from build123d import *

# Parameters (mm, degrees)
F0_R        = 15
F1_DEPTH    = 10.5
F3_R        = 0.75
F5_R        = 1
F6_T1_DEPTH = 20.8553390593


# Not quite as in the source:
# - a fillet or chamfer that OpenCascade refuses, or shapes differently, is made with other operations: its cross-section is extruded or revolved along the edge and cut away or added


with BuildPart() as f1:
    # F0 (on Top) → F1 (new body)
    with BuildSketch(Plane.XY):
        Polygon((-11.5, -19.5), (11.5, -19.5), (19.5, -11.5), (19.5, 11.5), (11.5, 19.5), (-11.5, 19.5), (-19.5, 11.5), (-19.5, -11.5), align=None)
        Circle(F0_R, mode=Mode.SUBTRACT)
    extrude(amount=F1_DEPTH)

    # F4: sweep along a path in F2
    with BuildLine(Plane.XY.offset(10.5)) as f4_path:
        Line((18.75, 11.1893398282), (18.75, -11.1893398282))
        Line((18.75, -11.1893398282), (11.1893398282, -18.75))
        Line((11.1893398282, -18.75), (-11.1893398282, -18.75))
        Line((-11.1893398282, -18.75), (-18.75, -11.1893398282))
        Line((-18.75, -11.1893398282), (-18.75, 11.1893398282))
        Line((-18.75, 11.1893398282), (-11.1893398282, 18.75))
        Line((-11.1893398282, 18.75), (11.1893398282, 18.75))
        Line((11.1893398282, 18.75), (18.75, 11.1893398282))
    # F3 (on Front) → F4 (sweep)
    with BuildSketch(Plane.XZ):
        with Locations((18.75, 10.5)):
            Circle(F3_R)
    sweep(path=f4_path.line, transition=Transition.RIGHT)

    # F5
    f5_edges = [f1.edges().sort_by_distance(p)[0] for p in [
        (18, 0, 10.5),
        (14.43934, -14.43934, 10.5),
        (0, -18, 10.5),
        (-14.43934, -14.43934, 10.5),
        (-18, 0, 10.5),
        (-14.43934, 14.43934, 10.5),
        (0, 18, 10.5),
        (14.43934, 14.43934, 10.5),
    ]]
    fillet(f5_edges, radius=F5_R)

    # F6: fillet of radius 5 on 8 edges, made by hand

    # F6_s2 → F6_t1 (cut)
    with BuildSketch(Plane.XY.offset(-5.1776695297)):
        with BuildLine():
            ThreePointArc((-18.0355339059, -12.9644660941), (-19.1193976626, -11.34234935), (-19.5, -9.4289321881))
            Line((-19.5, -9.4289321881), (-19.5, -11.5))
            Line((-19.5, -11.5), (-18.0355339059, -12.9644660941))
        make_face()
        with BuildLine():
            ThreePointArc((-9.4289321881, -19.5), (-11.34234935, -19.1193976626), (-12.9644660941, -18.0355339059))
            Line((-12.9644660941, -18.0355339059), (-11.5, -19.5))
            Line((-11.5, -19.5), (-9.4289321881, -19.5))
        make_face()
        with BuildLine():
            ThreePointArc((9.4289321881, -19.5), (11.34234935, -19.1193976626), (12.9644660941, -18.0355339059))
            Line((12.9644660941, -18.0355339059), (11.5, -19.5))
            Line((11.5, -19.5), (9.4289321881, -19.5))
        make_face()
        with BuildLine():
            ThreePointArc((18.0355339059, -12.9644660941), (19.1193976626, -11.34234935), (19.5, -9.4289321881))
            Line((19.5, -9.4289321881), (19.5, -11.5))
            Line((19.5, -11.5), (18.0355339059, -12.9644660941))
        make_face()
        with BuildLine():
            ThreePointArc((-9.4289321881, 19.5), (-11.34234935, 19.1193976626), (-12.9644660941, 18.0355339059))
            Line((-12.9644660941, 18.0355339059), (-11.5, 19.5))
            Line((-11.5, 19.5), (-9.4289321881, 19.5))
        make_face()
        with BuildLine():
            ThreePointArc((-19.5, 9.4289321881), (-19.1193976626, 11.34234935), (-18.0355339059, 12.9644660941))
            Line((-18.0355339059, 12.9644660941), (-19.5, 11.5))
            Line((-19.5, 11.5), (-19.5, 9.4289321881))
        make_face()
        with BuildLine():
            ThreePointArc((12.9644660941, 18.0355339059), (11.34234935, 19.1193976626), (9.4289321881, 19.5))
            Line((9.4289321881, 19.5), (11.5, 19.5))
            Line((11.5, 19.5), (12.9644660941, 18.0355339059))
        make_face()
        with BuildLine():
            ThreePointArc((19.5, 9.4289321881), (19.1193976626, 11.34234935), (18.0355339059, 12.9644660941))
            Line((18.0355339059, 12.9644660941), (19.5, 11.5))
            Line((19.5, 11.5), (19.5, 9.4289321881))
        make_face()
    extrude(amount=F6_T1_DEPTH, mode=Mode.SUBTRACT)


solid = f1.part
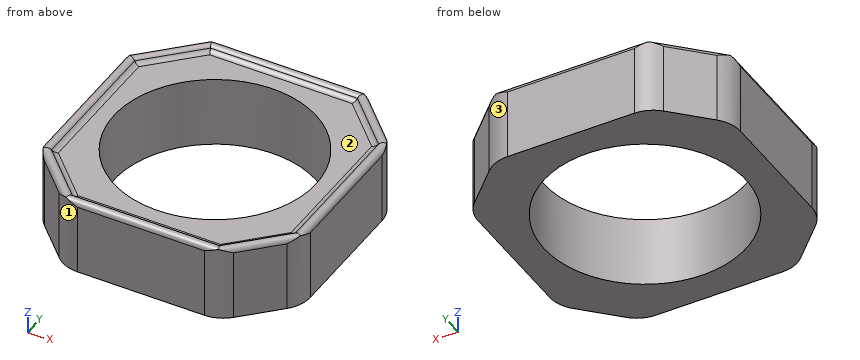
Source: CAD feature listing. Evaluate the final solid. Frame: model axes, mm. Face numbers are marked on the shaded views. Coordinates: 2 decimals unless noted, no trailing zeros. Loops run counter-clockwise (first coordinate to the right, second up) from the corner with the lowest first, then second, coordinate; pieces in that order, holes last. Notation, with made-up numbers: (-8.5, -33) -> (-3.5, -33) arc R30 ccw to (-3.5, 4) -> close; hole circle Ø2 at (30, -23.75). An arc over 180 degrees is marked (long way). Answer in a Markdown table with one row per item. Add a question column.
Q1. Contact query for flat-ended pins moving along their axis: pin 1 Ø3 at (x, y) = (11, 14.5) entering from +Z; pin 2 Ø1.5 at (y, z) = (13.5, 2.5) entering from -X; pin 3 Ø1 at (x, z) = (-10.5, 7) entering from -Y. Output: stop coordinate, or through.
Q2. Ray query, line 1 along Y through (x, z) = (0, 4.75); line 2 along Z through (x, y) = (11, -10.5); line 3 along X through (y, z) = (-7, 3). Return the intervals inside material, ascending.
Q3. Pull-direction query (X, two-part tool) for the marked faces 1, 2 and 3; classes: pulls with the +X half, pulls with the -X half, needs draft (parallel to the pull), parting line crosses it, or undercut.
Q4. Section C-C on z = 7.25. Return the cut outline in (x, y), and give its area (3 significant figures).
Q5. Section A-A on x = 0. Return the cut outline in (y, z), and give its area (3 significant figures).
Computed values:
| question | item | result |
|---|---|---|
| 1 | pin 1 | stops at z = 10.5 |
| 1 | pin 2 | stops at x = -18.24 |
| 1 | pin 3 | stops at y = -19.47 |
| 2 | line 1 | y = -19.5 to -15, 15 to 19.5 |
| 2 | line 2 | z = 0 to 10.5 |
| 2 | line 3 | x = -19.5 to -13.27, 13.27 to 19.5 |
| 3 | face 1 | pulls with the -X half |
| 3 | face 2 | undercut |
| 3 | face 3 | pulls with the +X half |
| 4 | outline | (-19.5, -9.43) arc R5 ccw to (-18.04, -12.96) -> (-12.96, -18.04) arc R5 ccw to (-9.43, -19.5) -> (9.43, -19.5) arc R5 ccw to (12.96, -18.04) -> (18.04, -12.96) arc R5 ccw to (19.5, -9.43) -> (19.5, 9.43) arc R5 ccw to (18.04, 12.96) -> (12.96, 18.04) arc R5 ccw to (9.43, 19.5) -> (-9.43, 19.5) arc R5 ccw to (-12.96, 18.04) -> (-18.04, 12.96) arc R5 ccw to (-19.5, 9.43) -> close; hole circle Ø30 at (0, 0) |
| 4 | area | 682 mm^2 |
| 5 | outline | (-19.5, 0) -> (-15, 0) -> (-15, 10.5) -> (-17.31, 10.5) arc R1 cw to (-18.13, 10.93) arc R0.75 ccw to (-19.5, 10.5) -> close; (15, 0) -> (19.5, 0) -> (19.5, 10.5) arc R0.75 ccw to (18.13, 10.93) arc R1 cw to (17.31, 10.5) -> (15, 10.5) -> close |
| 5 | area | 96.4 mm^2 |
